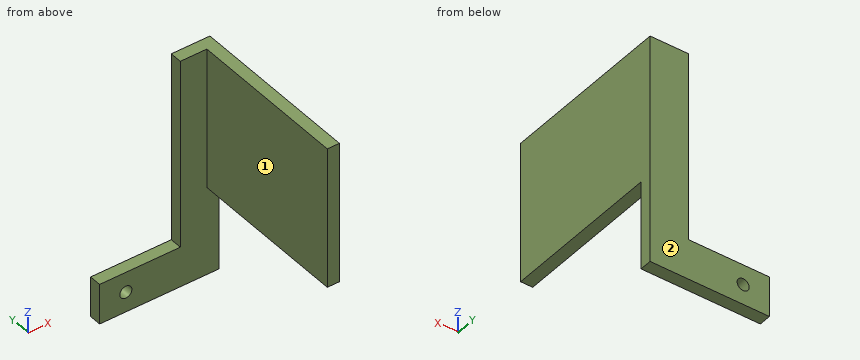
from build123d import *

# Parameters (mm, degrees)
BOSS_EXTRUDE1_DEPTH = 3
SKETCH2_R           = 1.5
CUT_EXTRUDE1_DEPTH  = 3
SKETCH3_W           = 3
SKETCH3_H           = 35
BOSS_EXTRUDE2_DEPTH = 40


with BuildPart() as part:
    # Sketch1 → Boss-Extrude1 (new body)
    with BuildSketch(Plane(origin=(0, 0, 0), x_dir=(1, 0, 0), z_dir=(0, 1, 0))):
        Polygon((10, -5), (10, -52), (19.57850172, -52), (19.57850172, 5), (10, 5), (-10, 5), (-10, -5), align=None)
    extrude(amount=BOSS_EXTRUDE1_DEPTH)

    # Sketch2 → Cut-Extrude1 (cut)
    with BuildSketch(Plane(origin=(0, 3, 0), x_dir=(1, 0, 0), z_dir=(0, 1, 0))):
        with Locations(Location((-3.5, 0, 0), (0, 0, 270))):
            Circle(SKETCH2_R)
    extrude(amount=-CUT_EXTRUDE1_DEPTH, mode=Mode.SUBTRACT)

    # Sketch3 → Boss-Extrude2 (add)
    with BuildSketch(Plane.XZ):
        with Locations((18.07850172, 34.5)):
            Rectangle(SKETCH3_W, SKETCH3_H)
    extrude(amount=BOSS_EXTRUDE2_DEPTH)


solid = part.part
Can you work these out from the model? Positions are in its coordinate system, mm. Face numbers are marked on the shaded views. A direction names the side the tool comes from. Give positions to 0.01 mm unless a question says otherwise; leave off trailing zeros. Loops run counter-clockwise (first coordinate to the right, second up) from the corner with the lowest first, then second, coordinate; pieces in that order, holes last. Notation, with made-up numbers: (-20, 45.25) - (-14, 45.25) arc R24 ccw to (-14, 83.25) - close; hole circle Ø7 at (-34, -29.5). An arc over 180 degrees is marked (long way). Answer as a JSON object with one key per item and string values.
Q1. Imagine slicing it at D-D on z = 23. Write out the boundary of the cut face in (x, y).
Geometry says:
{"outline": "(10, 0) - (16.58, 0) - (16.58, -40) - (19.58, -40) - (19.58, 3) - (10, 3) - close"}
Q2. Which directions (+Z, -Z, +X, -X, +Y, -Y) give clear straight access to the entire face, cutting with the end or side of a thin tool? Please do the marked faces 1 and 2.
Geometry says:
{"face 1": "+Z, -Z, -X, -Y", "face 2": "+Z, -Z, +X, -X, +Y"}
Q3. Imagine slicing it at A-A on x = -3.5. Write out the boundary of the cut face in (y, z).
Geometry says:
{"outline": "(0, -5) - (3, -5) - (3, -1.5) - (0, -1.5) - close; (0, 1.5) - (3, 1.5) - (3, 5) - (0, 5) - close"}
Q4. Imagine slicing it at C-C on y = -36. Write out the boundary of the cut face in (x, z).
Geometry says:
{"outline": "(16.58, 17) - (19.58, 17) - (19.58, 52) - (16.58, 52) - close"}
Q5. Will these pins go through, and if not, where does the flat tip stop? P1, Ø12, axis at y = -28, z = 6, coming from the -X side; P2, Ø1.5, axis at x = 10.5, z = 30.5, coming from the -Y side; P3, Ø2.5, axis at x = 18.5, y = -13.5, coming from the -Z side; P4, Ø0.9, axis at x = 3, y = 2, coming from the +Z side.
Geometry says:
{"P1": "through", "P2": "y = 0", "P3": "z = 17", "P4": "z = 5"}
Q6. If I drill on L1, parallel to X at y = 1, z = 0; L2, parallel to Y at x = 18.25, z = 4.5; L3, parallel to X at y = -23, z = 29, over which ranges is the centre line in solid material (lowest first)?
Geometry says:
{"L1": "-10 to -5, -2 to 19.58", "L2": "0 to 3", "L3": "16.58 to 19.58"}
Q7. Imagine slicing it at B-B on z = 0. Write out the boundary of the cut face in (x, y), plus the area to 3 significant figures.
Geometry says:
{"outline": "(-10, 0) - (-5, 0) - (-5, 3) - (-10, 3) - close; (-2, 0) - (19.58, 0) - (19.58, 3) - (-2, 3) - close", "area": "79.7 mm²"}
